Could you check a few things on this model? Use its own coordinates, in mm. Face numbers are marked on the shaded views. Coordinates: 2 decimals unless noted, no trailing zeros. Loops run counter-clockwise (first coordinate to the right, second up) from the corner with the lowest first, then second, coordinate; pieces in that order, holes last.
1) If I drill on line 1 along X through (y, z) = (93, -4); line 2 along Y through (x, z) = (-4.25, 5.75), over which ranges is the centre line in solid material (lowest first)?
2) Thinking about a two-plate mould opening in X: for the marked faces 1, 2, 3 and 4, which applies, released by +X, released by -X, zero draft, split by the parting line, or undercut?
3) Imagine slicing it at C-C on z = -1.5. Please give me the cut outline in (x, y).
4) Imagine slicing it at B-B on x = -2. Please give me the cut outline in (y, z).
5) Imagine slicing it at A-A on y = 183.5. Please give me the cut outline in (x, z).
```python
from build123d import *

# Parameters (mm, degrees)
SKETCH2_W               = 13
SKETCH2_H               = 13
SKETCH2_W_2             = 11
SKETCH2_H_2             = 11
BOSS_EXTRUDE1_DEPTH     = 240
CUT_EXTRUDE1_DEPTH      = 1
CUT_EXTRUDE1_DEPTH_BACK = 14
SKETCH4_OUTSIDE_W       = 63.14
SKETCH4_OUTSIDE_H       = 290.14
CUT_EXTRUDE2_DEPTH      = 240


with BuildPart() as part:
    # Sketch2 → Boss-Extrude1 (new body)
    with BuildSketch(Plane(origin=(0, 0, 0), x_dir=(1, 0, 0), z_dir=(0, 1, 0))):
        Rectangle(SKETCH2_W, SKETCH2_H)
        Rectangle(SKETCH2_W_2, SKETCH2_H_2, mode=Mode.SUBTRACT)
    extrude(amount=BOSS_EXTRUDE1_DEPTH)

    # Sketch3 → Cut-Extrude1 (cut, two sides)
    with BuildSketch(Plane.XY.offset(6.5)) as cut_extrude1_sk:
        Polygon((431.461827419, 485.351825456), (6.5, 240), (-6.5, 232.494446501), (-431.461827419, -12.857378955), (-922.165478331, 837.066275884), (-59.241823492, 1335.275480295), align=None)
    extrude(amount=CUT_EXTRUDE1_DEPTH, mode=Mode.SUBTRACT)
    extrude(cut_extrude1_sk.sketch, amount=-CUT_EXTRUDE1_DEPTH_BACK, mode=Mode.SUBTRACT)

    # Sketch4 outside → Cut-Extrude2 (cut)
    with BuildSketch(Plane.XY.offset(6.5)):
        with Locations((0, 120)):
            Rectangle(SKETCH4_OUTSIDE_W, SKETCH4_OUTSIDE_H)
        Polygon((6.5, 0), (-6.5, 7.505553499), (-6.5, 232.494446501), (6.5, 240), align=None, mode=Mode.SUBTRACT)
    extrude(amount=-CUT_EXTRUDE2_DEPTH, mode=Mode.SUBTRACT)


solid = part.part
```
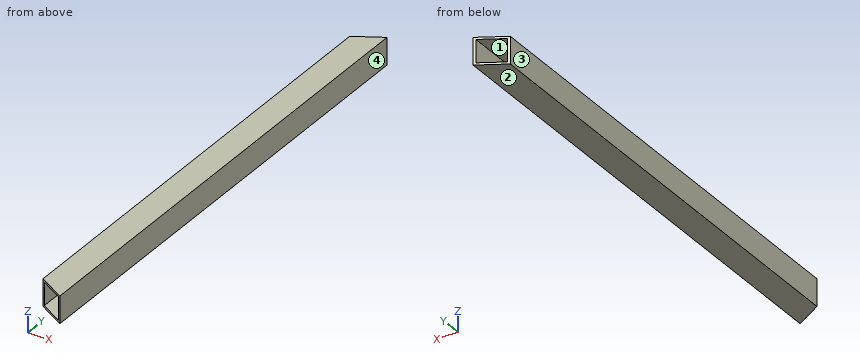
Filled in:
1. line 1: x = -6.5 to -5.5, 5.5 to 6.5
1. line 2: y = 6.21 to 233.79
2. face 1: undercut
2. face 2: zero draft
2. face 3: released by -X
2. face 4: released by +X
3. outline: (-6.5, 7.51) - (-5.5, 6.93) - (-5.5, 233.07) - (-6.5, 232.49) - close; (5.5, 0.58) - (6.5, 0) - (6.5, 240) - (5.5, 239.42) - close
4. outline: (4.91, -6.5) - (235.09, -6.5) - (235.09, -5.5) - (4.91, -5.5) - close; (4.91, 5.5) - (235.09, 5.5) - (235.09, 6.5) - (4.91, 6.5) - close
5. outline: (-6.5, -6.5) - (6.5, -6.5) - (6.5, 6.5) - (-6.5, 6.5) - close; hole (-5.5, -5.5) - (5.5, -5.5) - (5.5, 5.5) - (-5.5, 5.5) - close
